Geometry: see drawing. Coordinates: mm, zero at the bounding-box minimum. Round coordinates to 2 decimals unless told otherwise and drop trailing zeros. Loops run counter-clockwise (first coordinate to the right, second up) from the corner with the lowest first, then second, coordinate; pieces in that order, holes last.
(1) Section A-A, the plane x = 37.5. Return the cut outline in (y, z).
(2) Section C-C, the plane y = 135.5. Return the cut outline in (x, z), plus the area to 3 significant figures.
(3) Section D-D, the plane x = 54. Return the cut outline in (y, z).
(4) Section B-B, the plane z = 10.5. Return the cut outline in (x, y), plus the area to 3 significant figures.
(5) Material intervals for probe 1 along Y at (x, z) = (32, 12.75); probe 2 along Y at (x, z) = (59, 6.5); probe 3 along X at (y, z) = (293, 12.5), sorted ascending.
(6) First-contact query: pin 1 Ø6 at (x, y) = (12.5, 89.5) entering from -Z; pin 2 Ø1 at (y, z) = (176, 6) entering from -X; pin 3 Ø1.5 at (y, z) = (346.5, 5.5) entering from +X; pin 4 Ø6 at (x, z) = (12, 7) entering from +Y. Flat tips, straight axial feed; report the tip coordinate or a pass-through.
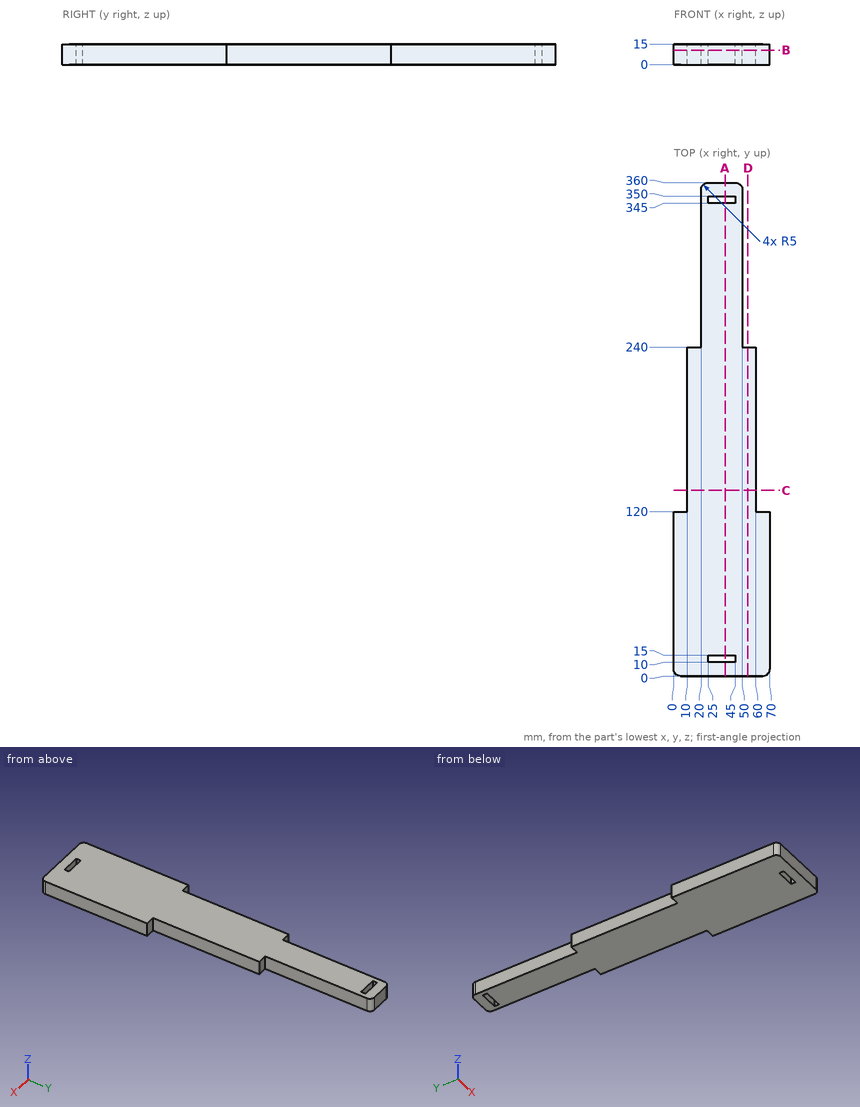
Output values:
1. outline: (0, 0) - (10, 0) - (10, 15) - (0, 15) - close; (15, 0) - (345, 0) - (345, 15) - (15, 15) - close; (350, 0) - (360, 0) - (360, 15) - (350, 15) - close
2. outline: (10, 0) - (60, 0) - (60, 15) - (10, 15) - close
2. area: 750 mm2
3. outline: (0, 0) - (240, 0) - (240, 15) - (0, 15) - close
4. outline: (0, 5) arc R5 ccw to (5, 0) - (65, 0) arc R5 ccw to (70, 5) - (70, 120) - (60, 120) - (60, 240) - (50, 240) - (50, 355) arc R5 ccw to (45, 360) - (25, 360) arc R5 ccw to (20, 355) - (20, 240) - (10, 240) - (10, 120) - (0, 120) - close; hole (25, 10) - (45, 10) - (45, 15) - (25, 15) - close; hole (25, 345) - (45, 345) - (45, 350) - (25, 350) - close
4. area: 17,800 mm2
5. probe 1: y = 0 to 10, 15 to 345, 350 to 360
5. probe 2: y = 0 to 240
5. probe 3: x = 20 to 50
6. pin 1: stops at z = 0
6. pin 2: stops at x = 10
6. pin 3: stops at x = 50
6. pin 4: stops at y = 240
